Autodesk Inventor part; units mm, degrees
ref_plane "YZ Plane" through (0, 0, 0) normal (1, 0, 0) x (0, 1, 0)
ref_plane "XZ Plane" through (0, 0, 0) normal (0, 1, 0) x (-1, 0, 0)
ref_plane "XY Plane" through (0, 0, 0) normal (0, 0, 1) x (1, 0, 0)
ref_plane "Work Plane1" through (122.7733, 133.3708, 9.0922) normal (0, 0, 1) x (1, 0, 0)
sketch "Sketch1" plane through (122.7733, 133.3708, 9.0922) normal (0, 0, 1) x (1, 0, 0)
  line L0 (-23.375, 1.75) -> (-8.375, 1.75) construction
  line L1 (-8.375, -214.25) -> (-23.375, -214.25) construction
  line L2 (-23.375, 1.75) -> (84.575, 1.75)
  line L3 (90.925, -4.6) -> (90.925, -207.9)
  line L4 (84.575, -214.25) -> (-23.375, -214.25)
  arc A0 (90.925, -4.6) -> (84.575, 1.75) centre (84.575, -4.6) ccw
  arc A1 (84.575, -214.25) -> (90.925, -207.9) centre (84.575, -207.9) ccw
  point P0 (-122.7733, -133.3708)
  point P1 (90.925, 1.75)
  point P2 (90.925, -214.25)
  dimension "d0" = 114.3
  dimension "d3" = 6.35
ref_plane "Work Plane3" through (99.3983, 135.1208, 9.0922) normal (-1, 0, 0) x (0, 1, 0)
ref_plane "Work Plane2" through (44.8233, 115.6208, -3.6078) normal (-1, 0, 0) x (0, 1, 0)
sketch "Sketch3" plane through (99.3983, 135.1208, 9.0922) normal (-1, 0, 0) x (0, 1, 0)
  line L0 (3.175, -9.525) -> (0, -9.525)
  line L1 (0, -9.525) -> (0, 9.525)
  line L2 (0, 9.525) -> (3.175, 9.525)
  line L3 (3.175, 9.525) -> (3.175, -9.525)
  line L4 (0, 7.5) -> (0, -7.5)
  line L5 (-1.2141, 0) -> (3.175, 0) construction
  point P0 (-135.1208, 9.0922)
  point P1 (0, 0)
  dimension "d4" = 3.175
  dimension "d15" = 19.05
sweep "Sweep1" add profiles "Sketch3" path "Sketch1"
fillet "Fillet1" radius 7.5 4 edges at (99.3983, 136.7083, -0.4328) (99.3983, -82.4667, -0.4328) (99.3983, 136.7083, 18.6172) (99.3983, -82.4667, 18.6172)
sketch "Sketch4" plane through (207.3483, -84.0542, -0.4328) normal (0, -1, 0) x (1, 0, 0)
  circle A0 centre (-100.45, 9.525) radius 2.7559
  point P0 (-207.3483, 0.4328)
hole "Hole1" at (106.8983, -84.0542, 9.0922) direction (0, 1, 0) diameter 5.3086 depth 3.175
ref_plane "Work Plane4" through (207.3483, 27.1208, 18.6172) normal (0, 1, 0) x (1, 0, 0)
mirror "Mirror1" about plane through (207.3483, 27.1208, 18.6172) normal (0, 1, 0) of "Hole1"
properties part number "Pivoting Bracket"
CAD build for the part. Positions are in the model's coordinates, mm. A direction names the side the tool comes from. Round coordinates to 2 decimals unless told otherwise and drop trailing zeros. Order: outer loops, then holes, each group sorted by start corner. A loop starts at its lowest first (then second) coordinate and runs counter-clockwise, first axis right, second up. Notation, with made-up numbers: (54, -21.5) - (94, -21.5) arc R13 cw to (94, -2.5) - close; hole circle Ø3 at (17.5, 49). An arc over 180 degrees is marked (long way). Answer as CSV lines item,"result". Start each with the question number.
1. Saw through at B-B, the plane z = 4. Write the cut outline in (x, y) (3 decimals).
2. Pull direction Y, two halves, no side cores. Call faces 1 (the face through (214.157, -81.19, 8.959)), 2 (the face through (211.9, 133.2, 9.2)), 3 (the face through (215, 27, 18.617)): +Y half, -Y half, draft (parallel to the pull), parting line (faces both ways), or undercut.
3. Saw through at C-C, the plane y = 106. Write the cut outline in (x, z).
4. Drill centre lines: L1, parallel to Y at x = 168, z = 5.5; L2, parallel to Y at x = 211, z = 15.5; L3, parallel to X at y = -45.5, z = 6.25. Where is each one in solid material? Low to high. Write a range as [from, to].
5. Saw through at A-A, the plane x = 133.5. Write the cut outline in (y, z).
6. Pin check, flat tip, straight feed: pin 1 (8 mm diameter, centred on y = 38.5, z = 15, fed in from -X). Stop position of the tip, or through.
7. Tool access for faces 4 (the face through (154, 135.121, 9)), 5 (the face through (216.873, 26, 9)): list every direction of +Z, -Z, +X, -X, +Y, -Y with a clear straight run to the whole face (end or side of a thin tool).
Model answer:
1,outline,"(100.054, -84.054) - (207.348, -84.054) arc R9.525 ccw to (216.873, -74.529) - (216.873, 128.771) arc R9.525 ccw to (207.348, 138.296) - (100.054, 138.296) - (100.054, 135.121) - (207.348, 135.121) arc R6.35 cw to (213.698, 128.771) - (213.698, -74.529) arc R6.35 cw to (207.348, -80.879) - (100.054, -80.879) - close"
2,face 1,"-Y half"
2,face 2,"undercut"
2,face 3,"draft"
3,outline,"(213.7, -0.43) - (216.87, -0.43) - (216.87, 18.62) - (213.7, 18.62) - close"
4,L1,"y = [-84.05, -80.88], [135.12, 138.3]"
4,L2,"y = [-83.33, -79.72], [133.97, 137.57]"
4,L3,"x = [213.7, 216.87]"
5,outline,"(-84.05, -0.43) - (-80.88, -0.43) - (-80.88, 18.62) - (-84.05, 18.62) - close; (135.12, -0.43) - (138.3, -0.43) - (138.3, 18.62) - (135.12, 18.62) - close"
6,pin 1,"stops at x = 213.7"
7,face 4,"+Z, -Z, -X"
7,face 5,"+Z, -Z, +X, +Y, -Y"
